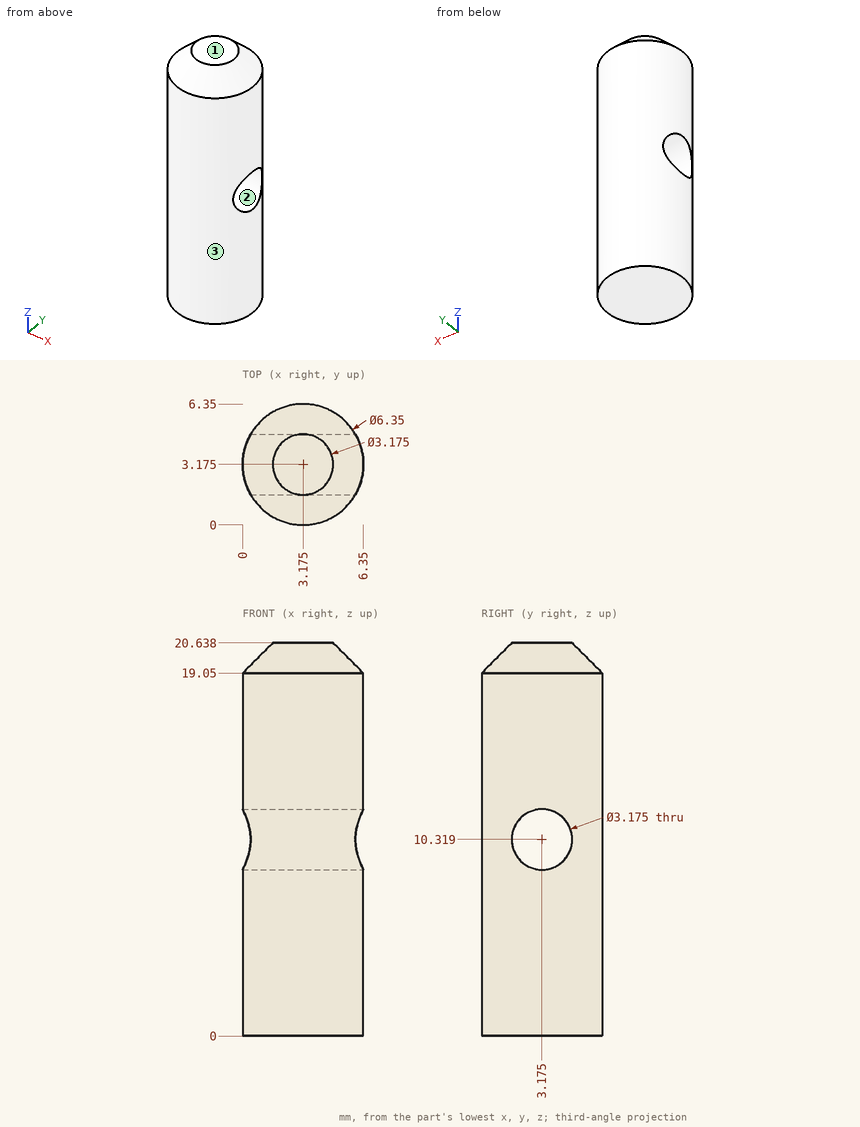
Verification items for this drawing (mm, ordinates from the low corner). Coordinates: 2 decimals unless noted, no trailing zeros. Put each result on its own line as item: value. Start each with the question number.
1. Go/stop test with a flat-tipped pin: pin 1 Ø2 at (x, z) = (2, 15.5) entering from -Y (1 decimal). Record where the tip stops, or that it passes through.
2. Mould release check, pull along Y, two halves, no side actions. Record for the marked faces 1, 2 and 3: released by +Y, released by -Y, zero draft, split by the parting line, or undercut.
3. Material ranges on L1, parallel to Y at x = 4, z = 10.5; L2, parallel to Y at x = 3.25, z = 5.25; L3, parallel to Z at x = 1, y = 4.5 (1 decimal), recorded low to high. Write a range as [from, to].
Computed:
1. pin 1: y = 0
2. face 1: zero draft
2. face 2: undercut
2. face 3: split by the parting line
3. L1: [0.11, 1.6], [4.75, 6.24]
3. L2: [0, 6.35]
3. L3: [0, 9.4], [11.2, 19.7]
